from build123d import *

# Parameters (mm, degrees)
SKETCH1_R           = 10
SKETCH1_R_2         = 3
BOSS_EXTRUDE1_DEPTH = 2
FILLET1_R           = 10
FILLET2_R           = 8
FILLET3_R           = 50


with BuildPart() as part:
    # Sketch1 → Boss-Extrude1 (new body)
    with BuildSketch(Plane.XY):
        with BuildLine():
            Line((-57.275649276, -30.405591591), (-28.125846456, -1.255788771))
            add(Edge.make_bspline(
                [(-28.125846456, -1.255788771), (-17.904305408, 22.543934761), (17.904305408, 22.543934761), (28.125846456, -1.255788771)],
                knots=[0, 0, 0, 0, 1, 1, 1, 1], degree=3))
            Line((28.125846456, -1.255788771), (57.275649276, -30.405591591))
            Line((57.275649276, -30.405591591), (30.405591591, -57.275649276))
            Line((30.405591591, -57.275649276), (0, -30))
            Line((0, -30), (-30.405591591, -57.275649276))
            Line((-30.405591591, -57.275649276), (-57.275649276, -30.405591591))
        make_face()
        Circle(SKETCH1_R, mode=Mode.SUBTRACT)
        with Locations((-42.426406871, -28.284271247)):
            Circle(SKETCH1_R_2, mode=Mode.SUBTRACT)
        with Locations((-28.284271247, -42.426406871)):
            Circle(SKETCH1_R_2, mode=Mode.SUBTRACT)
        with Locations((28.284271247, -42.426406871)):
            Circle(SKETCH1_R_2, mode=Mode.SUBTRACT)
        with Locations((42.426406871, -28.284271247)):
            Circle(SKETCH1_R_2, mode=Mode.SUBTRACT)
    extrude(amount=BOSS_EXTRUDE1_DEPTH)

    # Fillet1
    fillet1_edges = [part.edges().sort_by_distance(p)[0] for p in [
        (0, -30, 1),
    ]]
    fillet(fillet1_edges, radius=FILLET1_R)

    # Fillet2
    fillet2_edges = [part.edges().sort_by_distance(p)[0] for p in [
        (-57.275649276, -30.405591591, 1),
        (57.275649276, -30.405591591, 1),
        (30.405591591, -57.275649276, 1),
        (-30.405591591, -57.275649276, 1),
    ]]
    fillet(fillet2_edges, radius=FILLET2_R)

    # Fillet3
    fillet3_edges = [part.edges().sort_by_distance(p)[0] for p in [
        (-28.125846456, -1.255788771, 1),
        (28.125846456, -1.255788771, 1),
    ]]
    fillet(fillet3_edges, radius=FILLET3_R)


solid = part.part
Check sheet for the modelled part. Datum: model origin and axes. Units: mm. A direction names the side the tool comes from. Round coordinates to 2 decimals unless told otherwise and drop trailing zeros. Loops run counter-clockwise (first coordinate to the right, second up) from the corner with the lowest first, then second, coordinate; pieces in that order, holes last. Notation, with made-up numbers: (50, 42.5) -> (70, 42.5) arc R19 cw to (70, 70.5) -> close; hole circle Ø1 at (-23, -13). An arc over 180 degrees is marked (long way). Put each result on its own line as item: value. Start each with the question number.
1. Scan lines: probe 1 along Y at (x, z) = (0, 0.6); probe 2 along X at (y, z) = (-27, 0.55); probe 3 along X at (y, z) = (-40, 1.35). Record each from-to range of solid material in increasing order.
2. Section check C-C (z = 0.45). Give the number of separate pieces and of enclosed holes in the cut face, plus the area to 3 significant figures.
3. Section check A-A (y = -37.5). Enter the section's corners in (x, z).
4. Access from +Z, -Z, +X, -X, +Y, -Y to the whole of each face (thin tool, end or side, straight path). Record for faces 5 (the face through (-2.17, -9.76, 0.99)), 6 (the face through (-15.595, -43.989, 0.986)).
5. Section check B-B (y = -29.5). Enter the section's corners in (x, z).
6. Draft check along X on faces 1 (the face through (42.3, -15.43, 0.99)), 2 (the face through (-53.96, -30.49, 1.01)), 3 (the face through (15.85, -44.22, 0.99)), 4 (the face through (31.146, -41.525, 0.986)). Enter one of: +X half, -X half, draft (parallel to the pull), parting line (faces both ways), or undercut.
Findings:
1. probe 1: y = -33.43 to -10, 10 to 16.59
1. probe 2: x = -53.2 to -45.14, -39.72 to 39.72, 45.14 to 53.2
1. probe 3: x = -47.68 to -30.05, -26.52 to -11.15, 11.15 to 26.52, 30.05 to 47.68
2. separate pieces: 1
2. enclosed holes: 5
2. area: 4,290 mm^2
3. outline: (-50.18, 0) -> (-8.36, 0) -> (-8.36, 2) -> (-50.18, 2) -> close; (8.36, 0) -> (50.18, 0) -> (50.18, 2) -> (8.36, 2) -> close
4. face 5: +Z, -Z
4. face 6: +Z, -Z, -Y
5. outline: (-53.91, 0) -> (-45.17, 0) -> (-45.17, 2) -> (-53.91, 2) -> close; (-39.68, 0) -> (39.68, 0) -> (39.68, 2) -> (-39.68, 2) -> close; (45.17, 0) -> (53.91, 0) -> (53.91, 2) -> (45.17, 2) -> close
6. face 1: +X half
6. face 2: -X half
6. face 3: undercut
6. face 4: undercut
